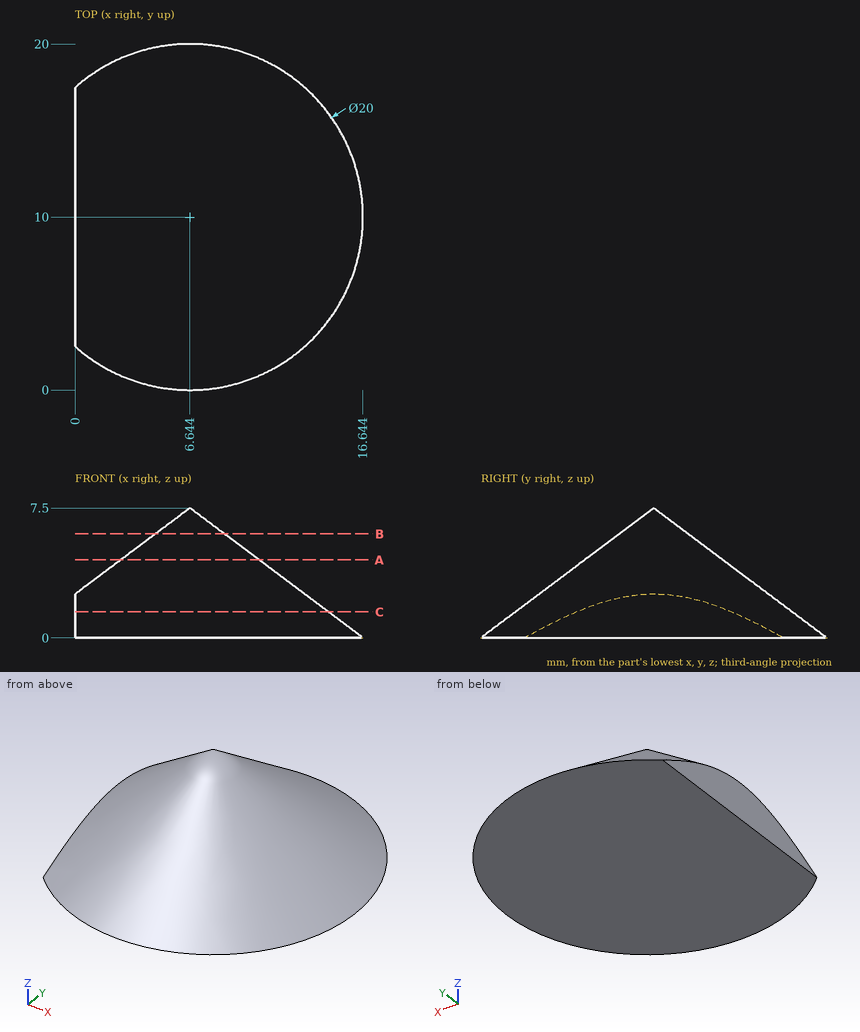
Check sheet for the drawn part. Datum: minimum x, y, z corner. Units: mm. Give positions to 0.01 mm unless a question says otherwise; leave off trailing zeros. Loops run counter-clockwise (first coordinate to the right, second up) from the corner with the lowest first, then second, coordinate; pieces in that order, holes last. Notation, with made-up numbers: M 73.25,84.25 L 96.25,84.25 A23 cw 96.25,98.25 Z; hole C 64.5,44 d2. An arc over 180 degrees is marked long. Return JSON: item names as keys, results as strings.
1) Section check C-C, the plane z = 1.5. Enter the section's corners in (x, y), and give its area (3 significant figures).
Findings:
{"outline": "M 0,5.54 A8 ccw long 0,14.46 Z", "area": "193 mm2"}
2) Section check B-B, the plane z = 6. Enter the section's corners in (x, y).
Findings:
{"outline": "C 6.64,10 d4"}
3) Material ranges on L1, parallel to Y at x = 8, z = 1.5 (1 decimal); L2, parallel to Z at x = 14.5, y = 13; L3, parallel to X at y = 14.5, z = 1, recorded low to high. Write a range as [from, to].
Findings:
{"L1": "y = [2.1, 17.9]", "L2": "z = [0, 1.19]", "L3": "x = [0, 14.05]"}
4) Section check A-A, the plane z = 4.5. Enter the section's corners in (x, y).
Findings:
{"outline": "C 6.64,10 d8"}
5) Gauge pin test, flat ends, axial feed: P1, Ø8, axis at x = 12, y = 17, coming from the +Z side; P2, Ø1, axis at y = 13, z = 1, coming from the +X side; P3, Ø2, axis at y = 4, z = 5, coming from the -X side. Record the tip position at first contact, or that the pin passes through.
Findings:
{"P1": "stops at z = 3.89", "P2": "stops at x = 15.5", "P3": "passes through"}
